Build history of the part. All positions in model axes, mm. Face numbers are marked on the shaded views. Round coordinates to 2 decimals unless told otherwise and drop trailing zeros. Loops run counter-clockwise (first coordinate to the right, second up) from the corner with the lowest first, then second, coordinate; pieces in that order, holes last.
from build123d import *

# Parameters (mm, degrees)
STOCK_RECORD_START          = -3.175
STOCK_RECORD_NEEDLE_1_DEPTH = 3.175
FILLET1_R                   = 3.175
NEEDLE_HOLE_DEPTH           = 157.399949281


# Read off the part's stored shape, not the designer's step: Stock-Record Needle-1
with BuildPart() as part:
    # Stock-Record Needle-1 outline → Stock-Record Needle-1 (new body)
    with BuildSketch(Plane(origin=(0, 0, 0), x_dir=(1, 0, 0), z_dir=(0, 1, 0)).offset(STOCK_RECORD_START)):
        Polygon((-134.794168142, 66.899467737), (-141.955930631, 60.428744281), (-141.955930631, 54.078744281), (-132.445850386, 43.348439368), (-122.158808708, 52.642883574), align=None)
    extrude(amount=STOCK_RECORD_NEEDLE_1_DEPTH)

    # Fillet1
    fillet1_edges = [part.edges().sort_by_distance(p)[0] for p in [
        (-132.445850386, -1.5875, -43.348439368),
        (-122.158808708, -1.5875, -52.642883574),
        (-134.794168142, -1.5875, -66.899467737),
        (-141.955930631, -1.5875, -60.428744281),
        (-141.955930631, -1.5875, -54.078744281),
    ]]
    fillet(fillet1_edges, radius=FILLET1_R)

    # Needle Hole Sketch → Needle Hole (cut, through all)
    with BuildSketch(Plane.XZ.offset(3.175)):
        Polygon((-136.903920332, -56.435895918), (-132.646865427, -51.72421007), (-130.291022503, -53.852737522), (-134.548077408, -58.564423371), align=None)
    extrude(amount=-NEEDLE_HOLE_DEPTH, mode=Mode.SUBTRACT)


solid = part.part
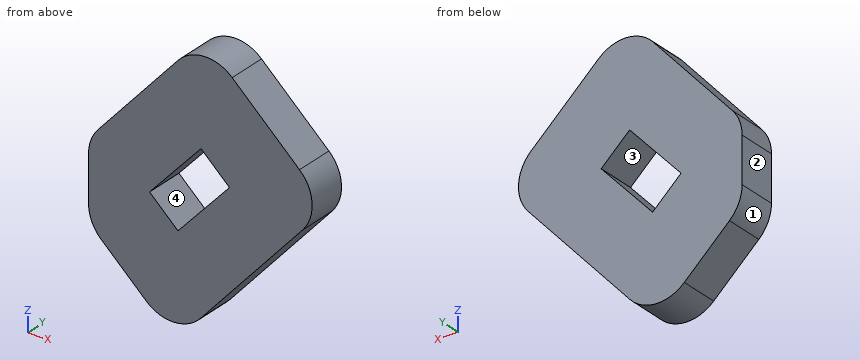
(1) Probe line 1 (X direction, y = -2.15, z = -57.75); line 2 (Z direction, x = -131.25, y = -1.6); line 3 (Z direction, x = -134.5, y = -2.6). List the from-to ranges inside material, lowest first.
Responses:
line 1: x = -141.96 to -135.45, -133.81 to -126.69
line 2: z = -62.9 to -54.91, -52.99 to -44.82
line 3: z = -65.52 to -58.51, -53.78 to -45.67
(2) Slice it at B-B on x = -135. List the corners of the cut face in (y, z) (3 decimals).
Responses:
outline: (-3.175, -65.569) - (0, -65.569) - (0, -58.156) - (-3.175, -58.156) - close; (-3.175, -54.329) - (0, -54.329) - (0, -46.23) - (-3.175, -46.23) - close
(3) Slice it at C-C on z = -54.75. List the corners of the cut face in (x, y) (3 decimals), plus the area to 3 significant figures.
Responses:
outline: (-141.911, -3.175) - (-135.381, -3.175) - (-135.381, 0) - (-141.911, 0) - close; (-131.102, -3.175) - (-124.047, -3.175) - (-124.047, 0) - (-131.102, 0) - close
area: 43.1 mm2
(4) Pin check, flat tip, straight feed: P1, Ø1, axis at x = -127, y = -0.5, coming from the -Z side. Stop position of the tip, or through.
Responses:
P1: stops at z = -58.67
(5) Slice it at D-D on x = -126.75. List the corners of the cut face in (y, z) (3 decimals), plus the area to 3 significant figures.
Responses:
outline: (-3.175, -57.823) - (0, -57.823) - (0, -48.495) - (-3.175, -48.495) - close
area: 29.6 mm2
(6) Pull direction Z, two halves, no side cores. Call the marked faces 1, 2, 3 and 4: +Z half, -Z half, draft (parallel to the pull), parting line (faces both ways), or undercut.
Responses:
face 1: -Z half
face 2: draft
face 3: undercut
face 4: undercut
(7) Slice it at A-A on y = -1.6. List the corners of the cut face in (x, z) (3 decimals).
Responses:
outline: (-141.956, -59.018) arc R3.175 ccw to (-140.909, -61.374) - (-137.173, -64.75) arc R3.175 ccw to (-132.668, -64.501) - (-124.245, -54.996) arc R3.175 ccw to (-124.492, -50.535) - (-130.067, -45.497) arc R3.175 ccw to (-134.572, -45.747) - (-141.157, -53.177) arc R3.175 ccw to (-141.956, -55.283) - close; hole (-136.904, -56.436) - (-134.548, -58.564) - (-130.291, -53.853) - (-132.647, -51.724) - close
